from build123d import *

# Parameters (mm, degrees)
F0_W      = 99.06
F0_H      = 78.74
F1_DEPTH  = 1.5748
F2_W      = 80.01
F2_H      = 35.8648
F3_DEPTH  = 7.62
F4_W      = 71.12
F4_H      = 24.13
F5_DEPTH  = 7.1628
F6_W      = 6.096
F6_H      = 6.096
F7_DEPTH  = 3.3782
F8_R      = 1.7145
F9_DEPTH  = 1.524
F10_R     = 1.524
F11_DEPTH = 12.7
F12_R     = 1.27
F13_W     = 6.858
F13_H     = 6.858
F14_DEPTH = 12.7
F15_R     = 1.4605
F16_DEPTH = 1.5748


with BuildPart() as f1:
    # F0 (on Top) → F1 (new body)
    with BuildSketch(Plane.XY):
        Rectangle(F0_W, F0_H)
    extrude(amount=F1_DEPTH)

    # F2 (on face) → F3 (join)
    with BuildSketch(Plane.XY.offset(1.5748)):
        with Locations((-3.6322, -19.7866)):
            Rectangle(F2_W, F2_H)
    extrude(amount=F3_DEPTH)

    # F4 (on face) → F5 (join)
    with BuildSketch(Plane.XY.offset(9.1948)):
        with Locations((-3.2512, -20.32)):
            Rectangle(F4_W, F4_H)
    extrude(amount=F5_DEPTH)

    # F6 (on face) → F7 (join)
    with BuildSketch(Plane.XY.offset(1.5748)):
        with Locations((43.307, -26.4668)):
            Rectangle(F6_W, F6_H)
        with Locations((43.307, -16.1798)):
            Rectangle(F6_W, F6_H)
        with Locations((43.307, -5.8928)):
            Rectangle(F6_W, F6_H)
    extrude(amount=F7_DEPTH)

    # F8 (on face) → F9 (join)
    with BuildSketch(Plane.XY.offset(4.953)):
        with Locations((43.307, -5.8928)):
            Circle(F8_R)
        with Locations((43.307, -16.1798)):
            Circle(F8_R)
        with Locations((43.307, -26.4668)):
            Circle(F8_R)
    extrude(amount=F9_DEPTH)

    # F10 (on face) → F11 (join)
    with BuildSketch(Plane.XY.offset(1.5748)):
        with Locations((6.604, 17.5514)):
            Circle(F10_R)
    extrude(amount=F11_DEPTH)

    # F12
    f12_edges = [f1.edges().sort_by_distance(p)[0] for p in [
        (5.08, 17.5514, 14.2748),
    ]]
    fillet(f12_edges, radius=F12_R)

    # F13 (on face) → F14 (join)
    with BuildSketch(Plane.XY.offset(1.5748)):
        with Locations((-25.146, 25.273)):
            Rectangle(F13_W, F13_H)
    extrude(amount=F14_DEPTH)

    # F15 (on face) → F16 (cut, through all)
    with BuildSketch(Plane(origin=(0, 0, 0), x_dir=(1, 0, 0), z_dir=(0, 0, -1))):
        with Locations((-46.99, 36.83)):
            Circle(F15_R)
        with Locations((45.085, 36.83)):
            Circle(F15_R)
        with Locations((45.085, -36.83)):
            Circle(F15_R)
        with Locations((-46.99, -36.83)):
            Circle(F15_R)
    extrude(amount=-F16_DEPTH, mode=Mode.SUBTRACT)


solid = f1.part
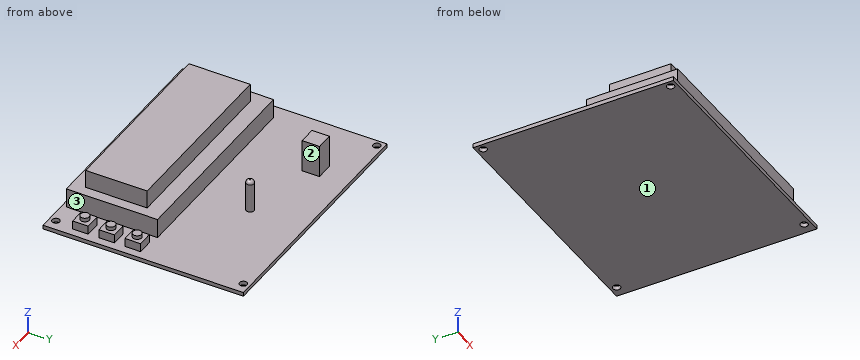
Read the model definition and answer for the solid it produces. Units are mm, in the model's axes. Face numbers are marked on the shaded views. A direction names the side the tool comes from. Coordinates: 2 decimals unless noted, no trailing zeros. Order: outer loops, then holes, each group sorted by start corner. A loop starts at its lowest first (then second) coordinate and runs counter-clockwise, first axis right, second up. Notation, with made-up numbers: (6.5, 3.25) - (35.5, 3.25) arc R13 ccw to (35.5, 22.25) - close; hole circle Ø11 at (-38.5, 40). An arc over 180 degrees is marked (long way). Use one line per item in the form item = value.
(1) Section D-D, the plane z = 2.75 is taken. Give the vertices of the cut face in (x, y) (3 decimals).
Computed values:
outline = (-43.637, -37.719) - (36.373, -37.719) - (36.373, -1.854) - (-43.637, -1.854) - close; (-28.575, 21.844) - (-21.717, 21.844) - (-21.717, 28.702) - (-28.575, 28.702) - close; circle Ø3.048 at (6.604, 17.551); (40.259, -29.515) - (46.355, -29.515) - (46.355, -23.419) - (40.259, -23.419) - close; (40.259, -19.228) - (46.355, -19.228) - (46.355, -13.132) - (40.259, -13.132) - close; (40.259, -8.941) - (46.355, -8.941) - (46.355, -2.845) - (40.259, -2.845) - close
(2) Straight lines are drawn through the part: L1, parallel to X at y = 36.83, z = 0.3; L2, parallel to Y at x = -46.99, z = 1; L3, parallel to X at y = -28.5, z = 10.25. For each, find the intervals that lie inside material, in ascending order.
Computed values:
L1 = -49.53 to -48.45, -45.53 to 43.62, 46.55 to 49.53
L2 = -39.37 to -38.29, -35.37 to 35.37, 38.29 to 39.37
L3 = -38.81 to 32.31
(3) Section A-A, the plane y = 36.83 is taken. Give the vertices of the cut face in (x, z).
Computed values:
outline = (-49.53, 0) - (-48.45, 0) - (-48.45, 1.57) - (-49.53, 1.57) - close; (-45.53, 0) - (43.62, 0) - (43.62, 1.57) - (-45.53, 1.57) - close; (46.55, 0) - (49.53, 0) - (49.53, 1.57) - (46.55, 1.57) - close
(4) Given pin 1 Ø5 at (x, y) = (44.5, -26.5) entering from +Z; pin 2 Ø5 at (y, z) = (-1, 9.5) entering from -X; pin 3 Ø7.5 at (y, z) = (27, 9.5) entering from -X (3 decimals), each flat-ended and moving along its own axis, determine where each tip first touches the part or whether it passes through.
Computed values:
pin_1 = 6.48
pin_2 = -43.64
pin_3 = -28.575
(5) Section C-C, the plane x = -46.99 is taken. Give the vertices of the cut face in (y, z).
Computed values:
outline = (-39.37, 0) - (-38.29, 0) - (-38.29, 1.57) - (-39.37, 1.57) - close; (-35.37, 0) - (35.37, 0) - (35.37, 1.57) - (-35.37, 1.57) - close; (38.29, 0) - (39.37, 0) - (39.37, 1.57) - (38.29, 1.57) - close
(6) Section B-B, the plane z = 10.75 is taken. Give the vertices of the cut face in (x, y) (3 decimals).
Computed values:
outline = (-38.811, -32.385) - (32.309, -32.385) - (32.309, -8.255) - (-38.811, -8.255) - close; (-28.575, 21.844) - (-21.717, 21.844) - (-21.717, 28.702) - (-28.575, 28.702) - close; circle Ø3.048 at (6.604, 17.551)
(7) Which of the six approach directions +Z, -Z, +X, -X, +Y, -Y give full straight-line access (tool end or side, diameter ignored) to the marked faces 1, 2 and 3?
Computed values:
face_1 = -Z, +X, -X, +Y, -Y
face_2 = +Z, +X, +Y
face_3 = +Z, +Y, -Y
